Verification items for the finished model (mm, model axes). Give positions to 0.01 mm unless a question says otherwise; leave off trailing zeros. Write each loop counter-clockwise with the first axis right and the second up, starting at its lowest first coordinate (ties: lowest second). Pieces come first, ordered by that corner, then holes. Notation, with made-up numbers: (15, 51.5) - (42, 51.5) arc R28 ccw to (42, 85.5) - close; hole circle Ø10 at (56.5, -17.75). An arc over 180 degrees is marked (long way). Put each result on its own line as item: value.
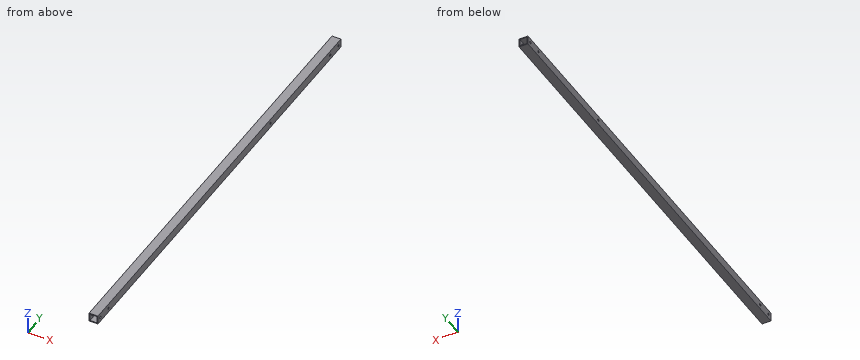
from build123d import *

# Parameters (mm, degrees)
SKETCH_1_W          = 15
SKETCH_1_H          = 15
SKETCH_1_W_2        = 12
SKETCH_1_H_2        = 12
EXTRUDE_1_DEPTH     = 741
SKETCH_2_R          = 2.1
SKETCH_2_R_2        = 2
CUT_EXTRUDE_1_DEPTH = 742.189753032


with BuildPart() as part:
    # ｽｹｯﾁ1 → 押し出し-薄板1 (new body)
    with BuildSketch(Plane(origin=(0, 0, 0), x_dir=(1, 0, 0), z_dir=(0, 1, 0))):
        Rectangle(SKETCH_1_W, SKETCH_1_H)
        Rectangle(SKETCH_1_W_2, SKETCH_1_H_2, mode=Mode.SUBTRACT)
    extrude(amount=EXTRUDE_1_DEPTH)

    # ｽｹｯﾁ2 → ｶｯﾄ - 押し出し1 (cut, through all)
    with BuildSketch(Plane(origin=(7.5, 0, 0), x_dir=(0, 0, -1), z_dir=(1, 0, 0))):
        with Locations((0, 7.29)):
            Circle(SKETCH_2_R)
        with Locations((0, 32.29)):
            Circle(SKETCH_2_R_2)
        with Locations((0, 708.71)):
            Circle(SKETCH_2_R_2)
        with Locations((0, 733.71)):
            Circle(SKETCH_2_R)
        with Locations((0, 526.49)):
            Circle(SKETCH_2_R)
    extrude(amount=-CUT_EXTRUDE_1_DEPTH, mode=Mode.SUBTRACT)


solid = part.part
Q1. Section check B-B, the plane x = -1.75. Record the cut outline in (y, z), plus the area to 3 significant figures.
Answers follow:
outline: (0, -7.5) - (741, -7.5) - (741, -6) - (0, -6) - close; (0, 6) - (741, 6) - (741, 7.5) - (0, 7.5) - close
area: 2,220 mm2
Q2. Section check A-A, the plane y = 201.5. Record the cut outline in (x, z), plus the area to 3 significant figures.
Answers follow:
outline: (-7.5, -7.5) - (7.5, -7.5) - (7.5, 7.5) - (-7.5, 7.5) - close; hole (-6, -6) - (6, -6) - (6, 6) - (-6, 6) - close
area: 81.0 mm2
Q3. Go/stop test with a flat-tipped pin: pin 1 Ø6.5 at (y, z) = (733.71, 0) entering from -X. Record where the tip stops, or that it passes through.
Answers follow:
pin 1: stops at x = -7.5
Q4. Scan lines: line 1 along Y through (x, z) = (6.45, 0); line 2 along Z through (x, y) = (-2, 280.5). Record each from-to range of solid material in increasing order.
Answers follow:
line 1: y = 0 to 5.19, 9.39 to 30.29, 34.29 to 524.39, 528.59 to 706.71, 710.71 to 731.61, 735.81 to 741
line 2: z = -7.5 to -6, 6 to 7.5
